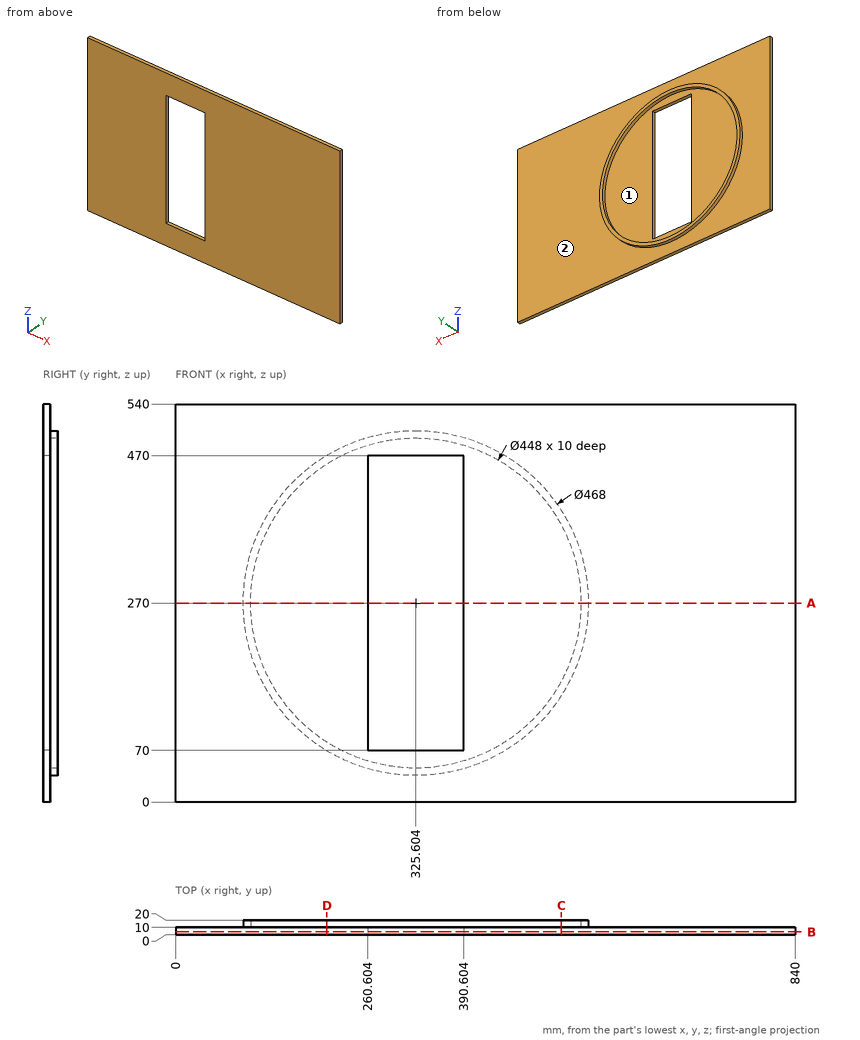
Study the drawing (mm; zero at the part's minimum x, y, z) and answer. Give positions to 0.01 mm unless a question says otherwise; leave off trailing zeros. Write each loop counter-clockwise with the first axis right and the second up, starting at its lowest first coordinate (ties: lowest second). Pieces come first, ordered by that corner, then holes. Notation, with made-up numbers: (32, -34) -> (63, -34) arc R17 ccw to (63, -3) -> close; hole circle Ø3 at (-40, -25.5). An arc over 180 degrees is marked (long way). Answer as a JSON object with one key per item and string values. Group by question number.
1) The mould has two halves that part along X. Classify the marked faces 1 and 2: +X half, -X half, draft (parallel to the pull), parting line (faces both ways), or undercut.
2) Consider L1, parallel to X at y = 9.5, z = 94; L2, parallel to X at y = 14.5, z = 270; L3, parallel to Y at x = 146, z = 396.5. Determine where each line is inside the solid, lowest interval first. Write a range as from..to.
3) Find section C-C (x = 523). Write down the section's boundary in (y, z).
4) Find section B-B (y = 4). Write down the section's boundary in (x, z), and give its area (3 significant figures).
5) Find section A-A (z = 270). Write down the section's boundary in (x, y), and give its area (3 significant figures).
6) Each of these flat-tipped pins is pushed along its axis until it touches: P1, Ø5, axis at x = 333.5, y = 4, coming from the -Z side; P2, Ø8, axis at x = 154.5, z = 473.5, coming from the +Y side; P3, Ø5, axis at x = 439, y = 13.5, coming from the -Z side; P4, Ø3, axis at y = 16, z = 396.5, coming from the +X side. Where does it stop, or does it pass through?
7) Find section D-D (x = 205). Write down the section's boundary in (y, z), and give its area (3 significant figures).
Values follow:
{
 "1": {"face 1": "undercut", "face 2": "draft"},
 "2": {"L1": "x = 0..260.6, 390.6..840", "L2": "x = 91.6..101.6, 549.6..559.6", "L3": "y = 0..10"},
 "3": {"outline": "(0, 0) -> (10, 0) -> (10, 144.34) -> (20, 144.34) -> (20, 164.12) -> (10, 164.12) -> (10, 375.88) -> (20, 375.88) -> (20, 395.66) -> (10, 395.66) -> (10, 540) -> (0, 540) -> close"},
 "4": {"outline": "(0, 0) -> (840, 0) -> (840, 540) -> (0, 540) -> close; hole (260.6, 70) -> (390.6, 70) -> (390.6, 470) -> (260.6, 470) -> close", "area": "402,000 mm2"},
 "5": {"outline": "(0, 0) -> (260.6, 0) -> (260.6, 10) -> (101.6, 10) -> (101.6, 20) -> (91.6, 20) -> (91.6, 10) -> (0, 10) -> close; (390.6, 0) -> (840, 0) -> (840, 10) -> (559.6, 10) -> (559.6, 20) -> (549.6, 20) -> (549.6, 10) -> (390.6, 10) -> close", "area": "7,300 mm2"},
 "6": {"P1": "stops at z = 0", "P2": "stops at y = 10", "P3": "stops at z = 63.95", "P4": "stops at x = 523.42"},
 "7": {"outline": "(0, 0) -> (10, 0) -> (10, 69.47) -> (20, 69.47) -> (20, 81.24) -> (10, 81.24) -> (10, 458.76) -> (20, 458.76) -> (20, 470.53) -> (10, 470.53) -> (10, 540) -> (0, 540) -> close", "area": "5,640 mm2"}
}
